Here's how the part is built. I have some questions about the finished solid (model axes, mm). Face numbers are marked on the shaded views. Round coordinates to 2 decimals unless told otherwise and drop trailing zeros. Order: outer loops, then holes, each group sorted by start corner. A loop starts at its lowest first (then second) coordinate and runs counter-clockwise, first axis right, second up. Notation, with made-up numbers: (8.5, 56) - (53.5, 56) arc R14 ccw to (53.5, 75) - close; hole circle Ø4 at (38.5, -31.5). An arc over 180 degrees is marked (long way). Answer as a JSON object with one key per item and string values.
```python
from build123d import *

# Parameters (mm, degrees)
SKETCH1_W           = 10
SKETCH1_H           = 12
BOSS_EXTRUDE1_DEPTH = 4.7625
SKETCH2_R           = 1.75
CUT_EXTRUDE1_DEPTH  = 12.7625
SKETCH4_W           = 1.501109308
SKETCH4_H           = 12
CUT_EXTRUDE2_DEPTH  = 1


with BuildPart() as part:
    # Sketch1 → Boss-Extrude1 (new body)
    with BuildSketch(Plane(origin=(0, 0, 0), x_dir=(1, 0, 0), z_dir=(0, 1, 0))):
        with Locations((5, 6)):
            Rectangle(SKETCH1_W, SKETCH1_H)
    extrude(amount=BOSS_EXTRUDE1_DEPTH)

    # Sketch2 → Cut-Extrude1 (cut)
    with BuildSketch(Plane.XY):
        with Locations((5, 2.38125)):
            Circle(SKETCH2_R)
    extrude(amount=-CUT_EXTRUDE1_DEPTH, mode=Mode.SUBTRACT)

    # Sketch4 → Cut-Extrude2 (cut)
    with BuildSketch(Plane(origin=(0, 4.7625, 0), x_dir=(1, 0, 0), z_dir=(0, 1, 0))):
        with Locations((5, 6)):
            Rectangle(SKETCH4_W, SKETCH4_H)
    extrude(amount=-CUT_EXTRUDE2_DEPTH, mode=Mode.SUBTRACT)


solid = part.part
```
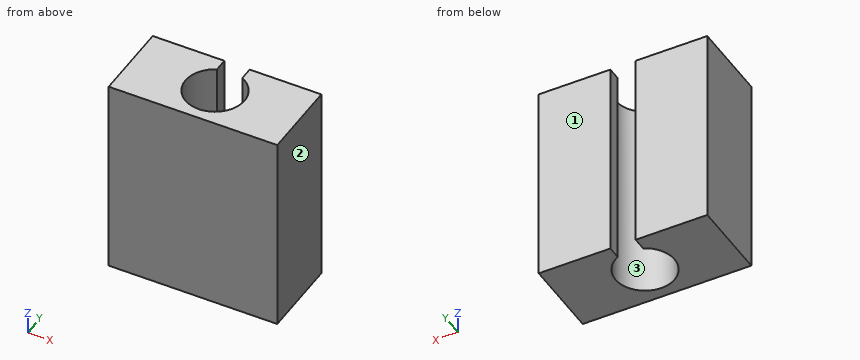
1. Imagine slicing it at A-A (z = -3.5). List the corners of the cut face in (x, y) for me.
Responses:
{"outline": "(0, 0) - (10, 0) - (10, 4.76) - (5.75, 4.76) - (5.75, 3.96) arc R1.75 cw (long way) to (4.25, 3.96) - (4.25, 4.76) - (0, 4.76) - close"}
2. Imagine slicing it at B-B (x = 5). List the corners of the cut face in (y, z) for me.
Responses:
{"outline": "(0, -12) - (0.63, -12) - (0.63, 0) - (0, 0) - close"}
3. Thinking about a two-plate mould opening in Y: for the marked faces 1, 2 and 3, which applies, pulls with the +Y half, pulls with the -Y half, needs draft (parallel to the pull), parting line crosses it, or undercut?
Responses:
{"face 1": "pulls with the +Y half", "face 2": "needs draft", "face 3": "undercut"}
4. For P1, Ø1.5, axis at y = 4, z = -3, coming from the -X side, with a flat end and sliding along its axis, tell me the tip position at first contact or that it passes through.
Responses:
{"P1": "x = 0"}
5. If I drill on L1, parallel to X at y = 2.45, z = -7.5; L2, parallel to X at y = 4.1, z = -9.5; L3, parallel to Y at x = 5, z = -6.75, over which ranges is the centre line in solid material (lowest first)? Write a range as [from, to].
Responses:
{"L1": "[0, 3.25], [6.75, 10]", "L2": "[0, 4.25], [5.75, 10]", "L3": "[0, 0.63]"}
